from build123d import *

# Parameters (mm, degrees)
SKETCH2_W           = 22.606
SKETCH2_H           = 12.192
BOSS_EXTRUDE2_DEPTH = 2.54
SKETCH3_W           = 10.16
SKETCH3_H           = 5.08
BOSS_EXTRUDE3_DEPTH = 15.24
SKETCH5_W           = 10.16
SKETCH5_H           = 7.62
BOSS_EXTRUDE4_DEPTH = 5.842
SKETCH6_W           = 5.08
SKETCH6_H           = 7.62
BOSS_EXTRUDE5_DEPTH = 35.56
SKETCH8_R           = 1.27
CUT_EXTRUDE2_DEPTH  = 5.08
CUT_EXTRUDE4_START  = -22.352
SKETCH4_R           = 0.635
CUT_EXTRUDE4_DEPTH  = 22.352
SKETCH16_W          = 10.16
SKETCH16_H          = 5.08
BOSS_EXTRUDE8_DEPTH = 6.35
SKETCH20_R          = 0.889
CUT_EXTRUDE7_DEPTH  = 3.556
SKETCH21_W          = 7.62
SKETCH21_H          = 5.08
BOSS_EXTRUDE9_DEPTH = 1.27


with BuildPart() as part:
    # Sketch2 → Boss-Extrude2 (new body)
    with BuildSketch(Plane.XY):
        Polygon((26.857381616, 17.540573563), (26.857381616, -4.811426437), (25.680950898, -4.811426437), (25.680950898, -42.911426437), (15.520950898, -42.911426437), (15.520950898, -4.811426437), (-10.988618384, -4.811426437), (-10.988618384, 17.540573563), (15.520950898, 17.540573563), (15.520950898, 55.640573563), (25.680950898, 55.640573563), (25.680950898, 17.540573563), align=None)
        with Locations((5.394381616, 6.364573563)):
            Rectangle(SKETCH2_W, SKETCH2_H, mode=Mode.SUBTRACT)
    extrude(amount=BOSS_EXTRUDE2_DEPTH)

    # Sketch3 → Boss-Extrude3 (add)
    with BuildSketch(Plane.XY.offset(2.54)):
        with Locations((-5.908618384, -2.271426437)):
            Rectangle(SKETCH3_W, SKETCH3_H)
    boss_extrude3 = extrude(amount=BOSS_EXTRUDE3_DEPTH)

    # Sketch5 → Boss-Extrude4 (add)
    with BuildSketch(Plane.XY.offset(2.54)):
        with Locations((20.600950898, -39.101426437)):
            Rectangle(SKETCH5_W, SKETCH5_H)
    boss_extrude4 = extrude(amount=BOSS_EXTRUDE4_DEPTH)

    # Sketch6 → Boss-Extrude5 (add)
    with BuildSketch(Plane.ZY.offset(-15.520950898)):
        with Locations((5.842, -39.101426437)):
            Rectangle(SKETCH6_W, SKETCH6_H)
    boss_extrude5 = extrude(amount=BOSS_EXTRUDE5_DEPTH)

    # Sketch8 → Cut-Extrude2 (cut)
    with BuildSketch(Plane.XY.offset(8.382)):
        with Locations((-14.959049102, -39.101426437)):
            Circle(SKETCH8_R)
    cut_extrude2 = extrude(amount=-CUT_EXTRUDE2_DEPTH, mode=Mode.SUBTRACT)

    # Mirror6: Boss-Extrude3, Boss-Extrude4, Boss-Extrude5, Cut-Extrude2 across plane
    add(boss_extrude3.mirror(Plane.ZX.offset(6.364573563)))
    add(boss_extrude4.mirror(Plane.ZX.offset(6.364573563)))
    add(boss_extrude5.mirror(Plane.ZX.offset(6.364573563)))
    add(cut_extrude2.mirror(Plane.ZX.offset(6.364573563)), mode=Mode.SUBTRACT)

    # Sketch4 → Cut-Extrude4 (cut)
    with BuildSketch(Plane(origin=(0, 17.540573563, 0), x_dir=(1, 0, 0), z_dir=(0, 1, 0)).offset(CUT_EXTRUDE4_START)):
        with Locations(Location((-5.908618384, -12.446, 0), (0, 0, 270))):
            Circle(SKETCH4_R)
    extrude(amount=CUT_EXTRUDE4_DEPTH, mode=Mode.SUBTRACT)

    # Sketch16 → Boss-Extrude8 (add)
    with BuildSketch(Plane(origin=(25.680950898, 0, 0), x_dir=(0, 0, -1), z_dir=(1, 0, 0))):
        with Locations((-5.08, -7.351426437)):
            Rectangle(SKETCH16_W, SKETCH16_H)
    extrude(amount=BOSS_EXTRUDE8_DEPTH)

    # Sketch20 → Cut-Extrude7 (cut)
    with BuildSketch(Plane(origin=(0, -9.891426437, 0), x_dir=(-1, 0, 0), z_dir=(0, -1, 0))):
        with Locations(Location((-28.982950898, -5.588, 0), (0, 0, 90))):
            Circle(SKETCH20_R)
    extrude(amount=-CUT_EXTRUDE7_DEPTH, mode=Mode.SUBTRACT)

    # Sketch21 → Boss-Extrude9 (add)
    with BuildSketch(Plane.ZY.offset(-25.680950898)):
        with Locations((6.35, -7.351426437)):
            Rectangle(SKETCH21_W, SKETCH21_H)
    extrude(amount=BOSS_EXTRUDE9_DEPTH)


solid = part.part
The listing builds one solid part. Answer for the finished solid, in the listing's coordinates (mm). A direction names the side the tool comes from. Round coordinates to 2 decimals unless told otherwise and drop trailing zeros. Write each loop counter-clockwise with the first axis right and the second up, starting at its lowest first coordinate (ties: lowest second). Pieces come first, ordered by that corner, then holes. Notation, with made-up numbers: (-1.5, 57.5) - (33.5, 57.5) arc R21 ccw to (33.5, 78.5) - close; hole circle Ø9 at (-19, 62). An arc over 180 degrees is marked (long way). Use one line per item in the form item = value. Start each with the question number.
Item 1: A cutting plane is placed at D-D (x = 23). Write down the section's boundary in (y, z), plus the area to 3 significant figures.
Item 2: A cutting plane is placed at A-A (y = 8.5). Write down the section's boundary in (x, z).
Item 3: A cutting plane is placed at C-C (x = -9.5). Write down the section's boundary in (y, z), plus the area to 3 significant figures.
Item 4: Flat-ended cylindrical pins translate along their axes: pin 1 Ø1.5 at (y, z) = (13, 3.5) entering from +X; pin 2 Ø4 at (y, z) = (-22.5, 4) entering from +X; pin 3 Ø8.5 at (x, y) = (1, 50) entering from -Z; pin 4 Ø4 at (y, z) = (43.5, 5) entering from +X. Find the tip coordinate at first contact, or state that the pin passes through.
Item 5: A cutting plane is placed at B-B (x = 7.5). Write down the section's boundary in (y, z), plus the area to 3 significant figures.
Item 6: A tool of negligible diameter and unlimited length cuts with its end or side. For faces 5 (the flat face through (3, -35.291, 5)), 6 (the flat face through (-3, 0.269, 7)), 7 (the flat face through (-4, -4.811, 9)), 8 (the flat face through (25.681, -30, 2)), 9 (the flat face through (-2, -39, 3.302)), from which of +Z, -Z, +X, -X, +Y, -Y can it reach the whole face along a straight path? Write none if from no direction.
Item 7: Determine the mould class of faces 1 (the flat face through (-5.909, 6, 1)), 2 (the flat face through (-20.039, 52, 6)), 3 (the flat face through (19, 7, 2.54)), 4 (the flat face through (16.697, 6, 1)) for opening direction X: +X half, -X half, draft (parallel to the pull), parting line (faces both ways), or undercut.
Item 8: Find the intervals of material crossed by line 1 (Y direction, x = -9.5, z = 6); line 2 (Y direction, x = 23.5, z = 5); line 3 (Y direction, x = -2, z = 15.5), in increasing order. Write a range as [from, to].
The answers:
q1.outline = (-42.91, 0) - (55.64, 0) - (55.64, 8.38) - (48.02, 8.38) - (48.02, 2.54) - (-35.29, 2.54) - (-35.29, 8.38) - (-42.91, 8.38) - close
q1.area = 339 mm^2
q2.outline = (-10.99, 0) - (-5.91, 0) - (-5.91, 2.54) - (-10.99, 2.54) - close; (16.7, 0) - (26.86, 0) - (26.86, 2.54) - (16.7, 2.54) - close
q3.outline = (-42.91, 3.3) - (-35.29, 3.3) - (-35.29, 8.38) - (-42.91, 8.38) - close; (-4.81, 0) - (17.54, 0) - (17.54, 17.78) - (12.46, 17.78) - (12.46, 2.54) - (0.27, 2.54) - (0.27, 17.78) - (-4.81, 17.78) - close; (48.02, 3.3) - (55.64, 3.3) - (55.64, 8.38) - (48.02, 8.38) - close
q3.area = 289 mm^2
q4.pin_1 = -0.83
q4.pin_2 = 25.68
q4.pin_3 = 3.3
q4.pin_4 = through
q5.outline = (-42.91, 3.3) - (-35.29, 3.3) - (-35.29, 8.38) - (-42.91, 8.38) - close; (-4.81, 0) - (0.27, 0) - (0.27, 2.54) - (-4.81, 2.54) - close; (12.46, 0) - (17.54, 0) - (17.54, 2.54) - (12.46, 2.54) - close; (48.02, 3.3) - (55.64, 3.3) - (55.64, 8.38) - (48.02, 8.38) - close
q5.area = 103 mm^2
q6.face_5 = +Z, +X, -X
q6.face_6 = +Z
q6.face_7 = +Z, -Z, -X
q6.face_8 = +Z, -Z, +X, -Y
q6.face_9 = -Z, -X, -Y
q7.face_1 = undercut
q7.face_2 = -X half
q7.face_3 = draft
q7.face_4 = undercut
q8.line_1 = [-42.91, -35.29], [-4.81, 0.27], [12.46, 17.54], [48.02, 55.64]
q8.line_2 = [-42.91, -35.29], [48.02, 55.64]
q8.line_3 = [-4.81, 0.27], [12.46, 17.54]
